For this review, use the dimensioned drawing (mm, ordinates from the lowest corner) and the shaded views. A direction names the side the tool comes from. Coordinates: 2 decimals unless noted, no trailing zeros. Order: outer loops, then holes, each group sorted by start corner. A loop starts at its lowest first (then second) coordinate and runs counter-clockwise, first axis right, second up. Notation, with made-up numbers: M -13.75,-10 L -3.75,-10 A29 cw -3.75,16 Z; hole C 78,69.5 d6. An arc over 180 degrees is marked long. Answer as CSV lines item,"result". Start each with the question number.
Q1. Consider section B-B on y = 1.7. Write out the cut boundary in (x, z), and give its area (3 significant figures).
Q2. The part is to be moulded in two halves that separate along X. For the marked faces 3, 4 and 5, say which applies: +X half, -X half, draft (parallel to the pull), parting line (faces both ways), or undercut.
Q3. Wall thickness on L1, parallel to Z at x = 2.5, y = 1.1; L2, parallel to Z at x = 2.5, y = 2.55; L3, parallel to Y at x = 8.5, z = 4: over which ranges is each line inside the solid? List them lowest first. Write a range as [from, to].
Q4. Consider section C-C on z = 3.5. Write out the cut boundary in (x, y).
Q5. For P1, Ø0.6, axis at y = 3, z = 1, coming from the -X side; P2, Ø1.5, axis at x = 2.5, z = 5.15, coming from the -Y side; P3, Ø2, axis at x = 1, y = 2, coming from the -Z side, all flat-tipped, find the tip position at first contact; note any pin that passes through.
Q6. Machinability: for the marked faces 1 and 2, which of the approach directions +Z, -Z, +X, -X, +Y, -Y give a long, thin tool a straight path to every point of the face, cutting with its end or side? Answer none if there is none.
Q7. Consider section D-D on y = 4.6. Write out the cut boundary in (x, z).
Q8. Consider section A-A on x = 5.75. Write out the cut boundary in (y, z).
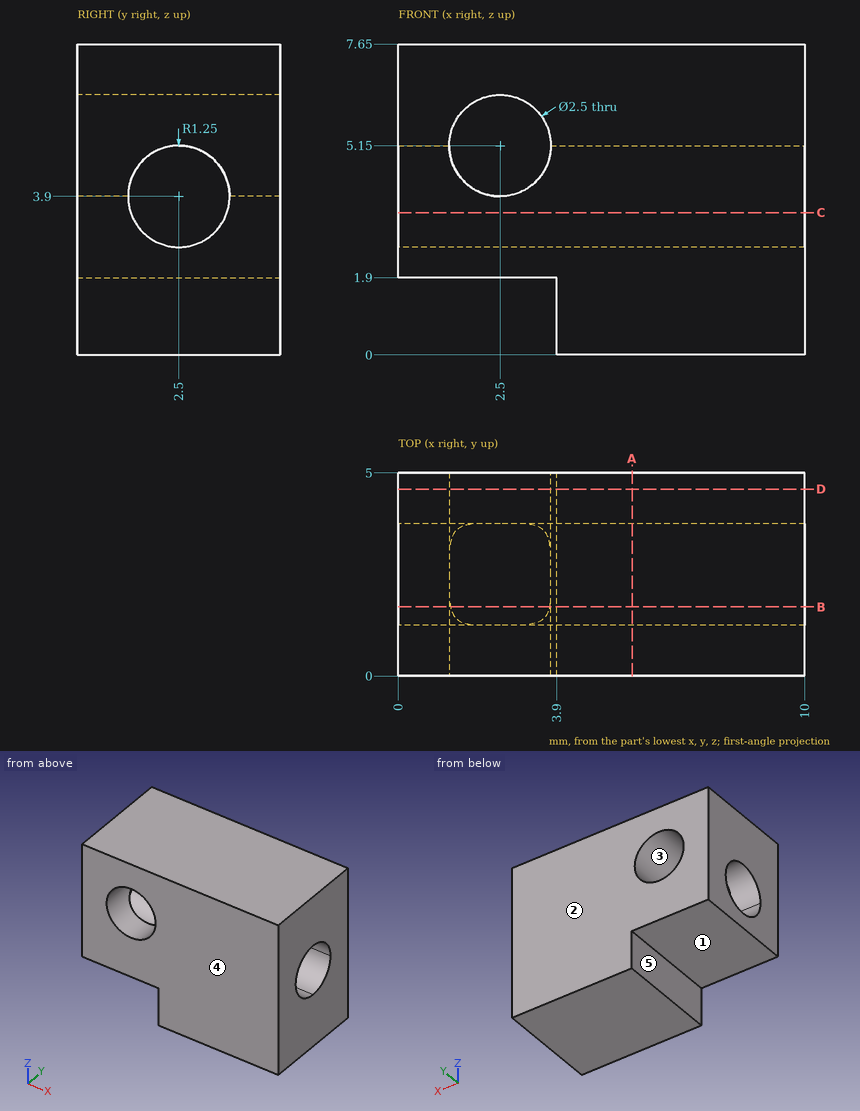
Evaluation:
1,outline,"M 0,1.9 L 3.9,1.9 L 3.9,0 L 10,0 L 10,2.94 L 0,2.94 Z; M 0,4.86 L 1.28,4.86 A1.25 cw long 3.72,4.86 L 10,4.86 L 10,7.65 L 0,7.65 Z"
1,area,"46.7 mm²"
2,face 3,"undercut"
2,face 4,"draft"
2,face 5,"-X half"
3,L1,"z = [1.9, 3.9], [6.4, 7.65]"
3,L2,"z = [1.9, 2.65], [6.4, 7.65]"
3,L3,"y = [0, 1.25], [3.75, 5]"
4,outline,"M 0,0 L 10,0 L 10,1.32 L 0,1.32 Z; M 0,3.68 L 10,3.68 L 10,5 L 0,5 Z"
5,P1,"stops at x = 3.9"
5,P2,"passes through"
5,P3,"stops at z = 1.9"
6,face 1,"-Z, -X, +Y, -Y"
6,face 2,"+Z, -Z, +X, -X, +Y"
7,outline,"M 0,1.9 L 3.9,1.9 L 3.9,0 L 10,0 L 10,7.65 L 0,7.65 Z; hole C 2.5,5.15 d2.5"
8,outline,"M 0,0 L 5,0 L 5,7.65 L 0,7.65 Z; hole C 2.5,3.9 d2.5"
